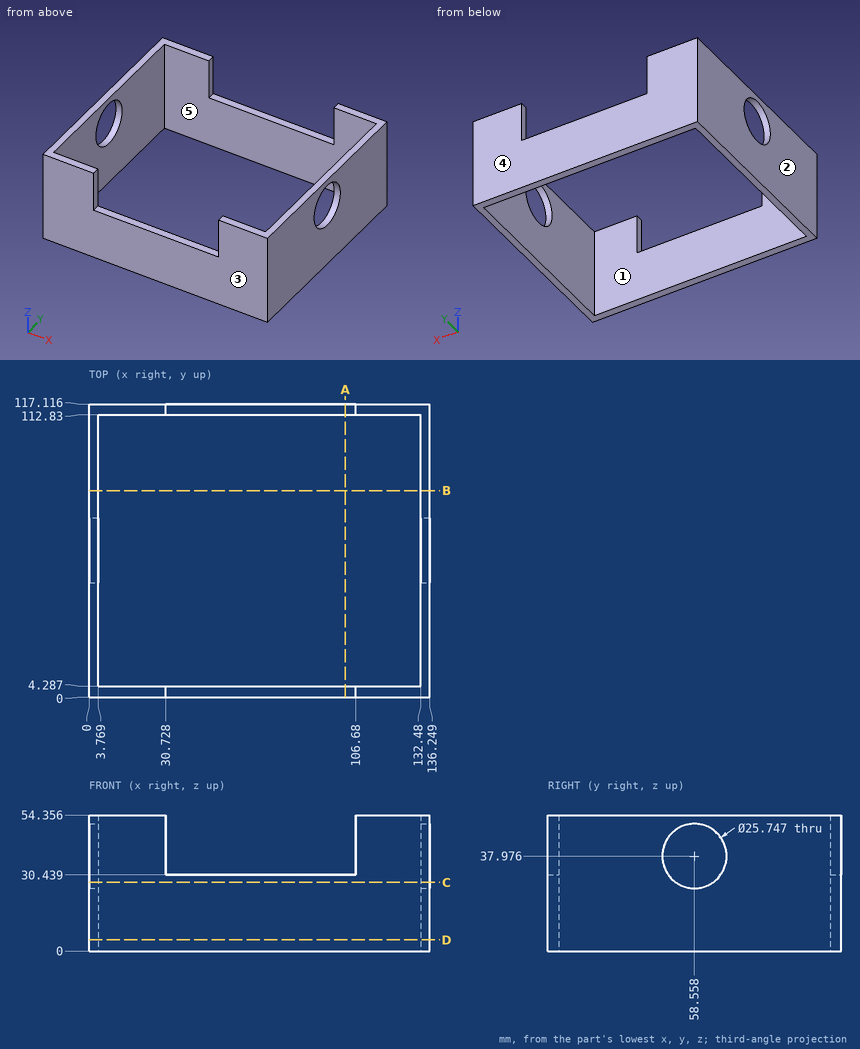
Answer from the drawing. Dimensions are ordinates in mm from the lowest x, y and z of the part. A direction names the side the tool comes from. Give positions to 0.01 mm unless a question says otherwise; leave off trailing zeros. Loops run counter-clockwise (first coordinate to the right, second up) from the corner with the lowest first, then second, coordinate; pieces in that order, holes last. Notation, with made-up numbers: (64, 61) - (75, 61) arc R34 cw to (75, 99) - close; hole circle Ø10 at (55.25, -19.75). An arc over 180 degrees is marked (long way). Answer as CSV lines item,"result". Start each with the question number.
Item 1: A cutting plane is placed at A-A on x = 102.5. Determine the outline of the cut face in (y, z).
Item 2: A cutting plane is placed at D-D on z = 4.5. Determine the outline of the cut face in (x, y), then the cut area to 3 significant figures.
Item 3: A cutting plane is placed at C-C on z = 27.5. Determine the outline of the cut face in (x, y), then the cut area to 3 significant figures.
Item 4: Find the intervals of material crossed by line 1 (Y direction, x = 43, z = 7); line 2 (X direction, y = 105.5, z = 34.5), in increasing order. Write a range as from..to.
Item 5: A cutting plane is placed at B-B on y = 82.5. Determine the outline of the cut face in (x, z).
Item 6: The mould has two halves that part along Y. Classify the marked faces 3, 4 and 5: +Y half, -Y half, draft (parallel to the pull), parting line (faces both ways), or undercut.
Item 7: This flat-tipped pin is pushed along its axis until it touches: pin 1 (4.5 mm diameter, centred on x = 62, y = 115, fed in from +Z). Where does it stop, or does it pass through?
Item 8: For the marked faces 1 and 2, determine the directions among +Z, -Z, +X, -X, +Y, -Y from which every point of the face is accessible in a straight line to the end or side of a thin tool.
Found:
1,outline,"(0, 0) - (4.29, 0) - (4.29, 30.44) - (0, 30.44) - close; (112.83, 0) - (117.12, 0) - (117.12, 30.44) - (112.83, 30.44) - close"
2,outline,"(0, 0) - (136.25, 0) - (136.25, 117.12) - (0, 117.12) - close; hole (3.77, 4.29) - (132.48, 4.29) - (132.48, 112.83) - (3.77, 112.83) - close"
2,area,"1,990 mm^2"
3,outline,"(0, 0) - (136.25, 0) - (136.25, 51.08) - (132.48, 51.08) - (132.48, 4.29) - (3.77, 4.29) - (3.77, 51.08) - (0, 51.08) - close; (0, 66.04) - (3.77, 66.04) - (3.77, 112.83) - (132.48, 112.83) - (132.48, 66.04) - (136.25, 66.04) - (136.25, 117.12) - (0, 117.12) - close"
3,area,"1,870 mm^2"
4,line 1,"y = 0..4.29, 112.83..117.12"
4,line 2,"x = 0..3.77, 132.48..136.25"
5,outline,"(0, 0) - (3.77, 0) - (3.77, 54.36) - (0, 54.36) - close; (132.48, 0) - (136.25, 0) - (136.25, 54.36) - (132.48, 54.36) - close"
6,face 3,"-Y half"
6,face 4,"+Y half"
6,face 5,"undercut"
7,pin 1,"stops at z = 30.44"
8,face 1,"+Z, -Z"
8,face 2,"+Z, -Z, -X, +Y, -Y"
